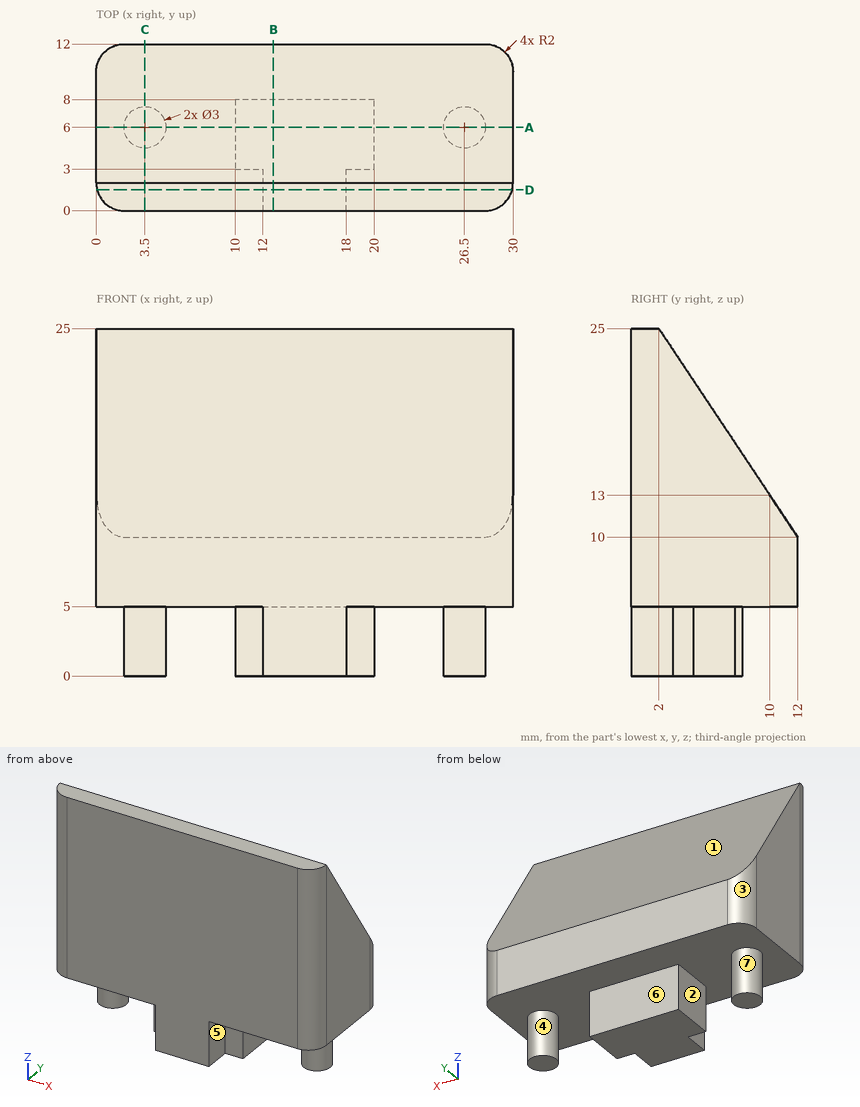
Geometry check sheet. Reference: drawing and pictorial views, mm from the part's lowest x, y, z. A direction names the side the tool comes from. Give positions to 0.01 mm unless a question says otherwise; leave off trailing zeros. Order: outer loops, then holes, each group sorted by start corner. A loop starts at its lowest first (then second) coordinate and runs counter-clockwise, first axis right, second up. Notation, with made-up numbers: M 25,-40 L 51,-40 A13 cw 51,-23 Z; hole C 39.25,86.5 d6. An arc over 180 degrees is marked long. Return JSON: item names as keys, results as strings. Group by question number.
1) Mould release check, pull along X, two halves, no side actions. Record for the marked faces 1, 2, 3 and 4: pulls with the +X half, pulls with the -X half, needs draft (parallel to the pull), parting line crosses it, or undercut.
2) Scan lines: line 1 (Z direction, x = 27.75, y = 1.75); line 2 (Y direction, x = 16.25, z = 20.5); line 3 (X direction, y = 1, z = 4.75). Record each from-to range of solid material in increasing order.
3) Section check C-C on x = 3.5. Record the cut outline in (y, z), and give its area (3 significant figures).
4) Go/stop test with flat-tipped pins: pin 1 Ø1.5 at (x, y) = (7, 3.5) entering from -Z; pin 2 Ø2.5 at (x, z) = (16.5, 1.5) entering from +Y; pin 3 Ø1.5 at (y, z) = (5.5, 3) entering from +X. Record where each tip stops, or that it passes through.
5) Access from +Z, -Z, +X, -X, +Y, -Y to the whole of each face (thin tool, end or side, straight path). Record for the marked faces 5, 6 and 7.
6) Section check D-D on y = 1.5. Record the cut outline in (x, z), and give its area (3 significant figures).
7) Section check A-A on y = 6. Record the cut outline in (x, z).
8) Section check B-B on x = 12.75. Record the cut outline in (y, z).
Answer block:
{
 "1": {"face 1": "needs draft", "face 2": "undercut", "face 3": "pulls with the -X half", "face 4": "undercut"},
 "2": {"line 1": "z = 5 to 25", "line 2": "y = 0 to 5", "line 3": "x = 12 to 18"},
 "3": {"outline": "M 0,5 L 4.5,5 L 4.5,0 L 7.5,0 L 7.5,5 L 12,5 L 12,10 L 2,25 L 0,25 Z", "area": "180 mm^2"},
 "4": {"pin 1": "stops at z = 5", "pin 2": "stops at y = 8", "pin 3": "stops at x = 28"},
 "5": {"face 5": "-Z, +X, -Y", "face 6": "-Z, +X, -X, +Y", "face 7": "-Z"},
 "6": {"outline": "M 0.06,5 L 12,5 L 12,0 L 18,0 L 18,5 L 29.94,5 L 29.94,25 L 0.06,25 Z", "area": "627 mm^2"},
 "7": {"outline": "M 0,5 L 2,5 L 2,0 L 5,0 L 5,5 L 10,5 L 10,0 L 20,0 L 20,5 L 25,5 L 25,0 L 28,0 L 28,5 L 30,5 L 30,19 L 0,19 Z"},
 "8": {"outline": "M 0,0 L 8,0 L 8,5 L 12,5 L 12,10 L 2,25 L 0,25 Z"}
}
